The listing builds one solid part. Answer for the finished solid, in the listing's coordinates (mm). Give positions to 0.01 mm unless a question says otherwise; leave off trailing zeros. Order: outer loops, then holes, each group sorted by start corner. A loop starts at its lowest first (then second) coordinate and runs counter-clockwise, first axis right, second up. Notation, with made-up numbers: (37, 58) - (65, 58) arc R21 cw to (65, 76) - close; hole circle Ø10 at (56, -37.5). An arc over 180 degrees is marked (long way). Answer as a JSON object with one key per item and string values. Group by question number.
Q1. A cutting plane is placed at A-A, the plane z = 0.35. Give the vertices of the cut face in (x, y).
Q2. A cutting plane is placed at C-C, the plane x = -12.5. Give the vertices of the cut face in (y, z).
Q3. A cutting plane is placed at B-B, the plane y = -7. Give the vertices of the cut face in (x, z), and give its area (3 significant figures).
Q4. A cutting plane is placed at D-D, the plane y = -16.5. Give the vertices of the cut face in (x, z), and give its area (3 significant figures).
Q5. Consider line 1 (X direction, y = -4, z = 0.4); line 2 (Y direction, x = -10, z = 0.2); line 3 (Y direction, x = 17.5, z = 0.15). Determine where each line is inside the solid, lowest interval first.
Autodesk Inventor part; units mm, degrees
ref_plane "XZ Plane" through (0, 0, 0) normal (0, 1, 0) x (-1, 0, 0)
sketch "Sketch1" plane through (0, 0, 0) normal (0, 0, 1) x (1, 0, 0)
  line L0 (-62, 19) -> (62, 19)
  line L1 (70, 11) -> (70, -11)
  line L2 (62, -19) -> (-62, -19)
  line L3 (-70, -11) -> (-70, 11)
  arc A0 (70, 11) -> (62, 19) centre (62, 11) ccw
  arc A1 (62, -19) -> (70, -11) centre (62, -11) ccw
  arc A2 (-70, -11) -> (-62, -19) centre (-62, -11) ccw
  arc A3 (-62, 19) -> (-70, 11) centre (-62, 11) ccw
  point P0 (0, 0)
  dimension "d0" = 19
  dimension "d1" = 38
  dimension "d2" = 140
  dimension "d3" = 70
  dimension "d4" = 8
  dimension "d5" = 8
extrude "Extrusion1" add sketch "Sketch1" along normal blind 0.5
sketch "Sketch2" plane through (0, 0, 0) normal (0, 0, 1) x (1, 0, 0)
  arc A0 (-49.9899, -19.1353) -> (-52, -19) centre (-52, -34) ccw
  arc A1 (52, -19) -> (49.9899, -19.1353) centre (52, -34) ccw
  line L0 (52, -17) -> (52, -19)
  line L1 (70, -11) -> (70, 11)
  line L2 (-70, 11) -> (-70, -11)
  line L3 (-62, -19) -> (62, -19)
  line L4 (-52, -34) -> (-52, -17)
  line L5 (-52, -17) -> (52, -17)
  line L6 (52, -17) -> (52, -19)
  arc A2 (-49.9899, -19.1353) -> (49.9899, -19.1353) centre (0, 350.5357) ccw
  dimension "d24" = 30
  dimension "d25" = 30
  dimension "d26" = 18
  dimension "d27" = 15
  dimension "d28" = 15
  dimension "d30" = 2
  dimension "d31" = 18
  dimension "d32" = 5.5
extrude "Extrusion2" add sketch "Sketch2" along normal blind 0.5
sketch "Sketch3" plane through (0, 0, 0) normal (0, 0, 1) x (1, 0, 0)
  arc A0 (62, -19) -> (70, -11) centre (62, -11) ccw
  arc A1 (-62, 19) -> (-70, 11) centre (-62, 11) ccw
  line L0 (-62, 11) -> (62, 11)
  line L1 (62, 11) -> (62, -11)
  line L2 (62, -11) -> (-62, -11)
  line L3 (-62, -11) -> (-62, 11)
  point P0 (0, 0)
extrude "Extrusion3" cut sketch "Sketch3" along normal through all both and the other way through all
properties part number "frontprofile"
Reply:
{
 "1": {"outline": "(-70, -11) arc R8 ccw to (-62, -19) - (-52, -19) arc R15 cw to (-49.99, -19.14) arc R373.04 ccw to (49.99, -19.14) arc R15 cw to (52, -19) - (62, -19) arc R8 ccw to (70, -11) - (70, 11) arc R8 ccw to (62, 19) - (-62, 19) arc R8 ccw to (-70, 11) - close; hole (-62, -11) - (62, -11) - (62, 11) - (-62, 11) - close"},
 "2": {"outline": "(-22.29, 0) - (-11, 0) - (-11, 0.5) - (-22.29, 0.5) - close; (11, 0) - (19, 0) - (19, 0.5) - (11, 0.5) - close"},
 "3": {"outline": "(-70, 0) - (-62, 0) - (-62, 0.5) - (-70, 0.5) - close; (62, 0) - (70, 0) - (70, 0.5) - (62, 0.5) - close", "area": "8.00 mm^2"},
 "4": {"outline": "(-67.81, 0) - (67.81, 0) - (67.81, 0.5) - (-67.81, 0.5) - close", "area": "67.8 mm^2"},
 "5": {"line 1": "x = -70 to -62, 62 to 70", "line 2": "y = -22.37 to -11, 11 to 19", "line 3": "y = -22.09 to -11, 11 to 19"}
}
